Here's how the part is built. I have some questions about the finished solid (model axes, mm). A direction names the side the tool comes from. Round coordinates to 2 decimals unless told otherwise and drop trailing zeros. Loops run counter-clockwise (first coordinate to the right, second up) from the corner with the lowest first, then second, coordinate; pieces in that order, holes last. Notation, with made-up numbers: M 38.25,18 L 51.25,18 A33 ccw 51.25,54 Z; hole C -8,32 d7. An arc over 180 degrees is marked long. Answer as a JSON object with one key per item and string values.
Autodesk Inventor part; units mm, degrees
ref_plane "Work Plane1" through (-10, 2, -13) normal (1, 0, 0) x (0, 0, -1)
ref_plane "Work Plane2" through (0, 0, -6.5) normal (0, 0, -1) x (-1, 0, 0)
ref_plane "Work Plane3" through (0, 0, 0) normal (1, 0, 0) x (0, 0, -1)
sketch "Sketch1" plane through (0, 0, 0) normal (0, 1, 0) x (-1, 0, 0)
  line L0 (0, 0) -> (-20, 0)
  line L1 (-20, 0) -> (-20, -13)
  line L2 (-20, -13) -> (0, -13)
  line L3 (0, -13) -> (0, 0)
  line L4 (0, -13) -> (20, -13)
  line L5 (20, -13) -> (20, -10)
  line L6 (20, -10) -> (0, -10)
  line L7 (0, -10) -> (0, -13)
  line L8 (0, -13) -> (-20, -13)
  line L9 (-20, -13) -> (-20, -23)
  line L10 (-20, -23) -> (0, -23)
  line L11 (0, -23) -> (0, -13)
  line L12 (20, -10) -> (0, -10)
  line L13 (0, -10) -> (0, 0)
  line L14 (0, 0) -> (20, 0)
  line L15 (20, 0) -> (20, -10)
  dimension "d0" = 20
  dimension "d1" = 13
  dimension "d2" = 20
  dimension "d3" = 3
  dimension "d4" = 10
extrude "Extrusion1" add sketch "Sketch1" along normal blind 2 contours L3 L2 L1 L0 | L2 L11 L10 L9
extrude "Extrusion2" add sketch "Sketch1" along normal blind 22 contours L6 L5 L4 L3
extrude "Extrusion3" add sketch "Sketch1" along normal blind 2 contours L14 L15 L6 L3
ref_plane "Work Plane1" through (-10, 2, -13) normal (1, 0, 0) x (0, 0, -1)
sketch "Sketch2" plane through (-10, 2, -13) normal (1, 0, 0) x (0, 0, -1)
  line L0 (0, 20) -> (-3, 20)
  line L1 (-13, -2) -> (-13, 0)
  line L2 (-13, 0) -> (-3, 0)
  line L3 (-3, 0) -> (-3, 20)
  line L4 (-3, 0) -> (-3, 20)
  line L5 (-3, 20) -> (-13, 20)
  line L6 (-13, 20) -> (-13, 0)
  line L7 (-13, 0) -> (-3, 0)
  line L8 (-3, 0) -> (-3, 20)
extrude "Extrusion4" add sketch "Sketch2" along normal mid plane 20
fillet "Fillet1" radius 10 1 edges at (-10, 22, 0)
sketch "Sketch3" plane through (0, 0, -13) normal (0, 0, -1) x (-1, 0, 0)
  circle A0 centre (10, 16) radius 1.5
  line L0 (0, 22) -> (20, 22)
  circle A1 centre (10, 6) radius 1.5
  line L1 (0, 0) -> (20, 0)
  point P0 (10, 0)
  dimension "d14" = 3
  dimension "d15" = 6
  dimension "d16" = 3
  dimension "d18" = 6
extrude "Extrusion5" cut sketch "Sketch3" against normal blind 20
ref_plane "Work Plane2" through (0, 0, -6.5) normal (0, 0, -1) x (-1, 0, 0)
sketch "Sketch4" plane through (0, 0, -6.5) normal (0, 0, -1) x (-1, 0, 0)
  circle A0 centre (10, 16) radius 1.5
  circle A1 centre (10, 16) radius 3
  circle A2 centre (10, 6) radius 1.5
  circle A3 centre (10, 6) radius 3
  point P0 (0, 0)
  dimension "d21" = 6
  dimension "d22" = 6
extrude "Extrusion6" cut sketch "Sketch4" against normal blind 20
sketch "Sketch5" plane through (0, 0, -13) normal (0, 0, -1) x (-1, 0, 0)
  line L0 (0, 22) -> (20, 22)
  line L1 (0, 0) -> (20, 0)
  line L2 (0, 22) -> (20, 22)
  line L3 (20, 22) -> (20, 0)
  line L4 (20, 0) -> (0, 0)
  line L5 (0, 0) -> (0, 22)
  circle A0 centre (10, 16) radius 1.5
  circle A1 centre (10, 16) radius 1.5
  circle A2 centre (10, 6) radius 1.5
  circle A3 centre (10, 6) radius 1.5
extrude "Extrusion7" add sketch "Sketch5" along normal blind 10
ref_plane "Work Plane3" through (0, 0, 0) normal (1, 0, 0) x (0, 0, -1)
sketch "Sketch6" plane through (0, 0, 0) normal (1, 0, 0) x (0, 0, -1)
  line L0 (0, 0) -> (23, 0)
  line L1 (23, 0) -> (23, -2)
  line L2 (23, -2) -> (0, 0)
  line L3 (0, 0) -> (23, 0)
  dimension "d27" = 2
extrude "Extrusion8" add sketch "Sketch6" along normal mid plane 40
sketch "Sketch7" plane through (0, 22, -23) normal (0, 0, -1) x (-1, 0, 0)
  line L0 (20, 0) -> (0, 0)
  line L1 (20, -24) -> (20, -22)
  line L2 (0, 0) -> (20, 0)
  line L3 (20, 0) -> (20, -24)
  line L4 (20, -24) -> (0, -24)
  line L5 (0, -24) -> (0, 0)
  line L6 (0, -20) -> (-20, -20)
  line L7 (-20, -20) -> (0, -20)
  line L8 (0, -20) -> (0, -24)
  line L9 (0, -24) -> (-20, -24)
  line L10 (-20, -24) -> (-20, -20)
  circle A0 centre (10, -6) radius 1.5
  circle A1 centre (10, -6) radius 1.5
  circle A2 centre (10, -16) radius 1.5
  circle A3 centre (10, -16) radius 1.5
  point P0 (0, -22)
extrude "Extrusion9" add sketch "Sketch7" along normal blind 10
sketch "Sketch8" plane through (0, 0, 0) normal (1, 0, 0) x (0, 0, -1)
  line L0 (23, -2) -> (33, -2)
  line L1 (33, -2) -> (33, -3)
  line L2 (33, -3) -> (23, -2)
  point P0 (0, 0)
  dimension "d32" = 1
extrude "Extrusion10" add sketch "Sketch8" along normal mid plane 40
sketch "Sketch9" plane through (20, 0, 0) normal (1, 0, 0) x (0, 0, -1)
  line L0 (33, 2) -> (0, 2)
  line L1 (0, 2) -> (33, 2)
  line L2 (33, 2) -> (33, -3)
  line L3 (33, 2) -> (33, -3)
  line L4 (23, -2) -> (0, 0)
  line L5 (33, -3) -> (0, 0)
  line L6 (0, 0) -> (0, 2)
extrude "Extrusion11" add sketch "Sketch9" along normal blind 10
sketch "Sketch10" plane through (0, 22, -33) normal (0, 0, -1) x (-1, 0, 0)
  line L0 (0, -20) -> (-30, -20)
  line L1 (-30, -20) -> (0, -20)
  line L2 (0, -20) -> (0, -25)
  line L3 (-20, -25) -> (20, -25)
  line L4 (-30, -25) -> (-30, -20)
  line L5 (-30, -25) -> (-30, -20)
  line L6 (-20, -24) -> (-20, -25)
  line L7 (-20, -25) -> (-30, -25)
  line L8 (-20, -25) -> (-30, -25)
  point P0 (0, -22)
extrude "Extrusion12" add sketch "Sketch10" along normal blind 9
properties part number "Holder Motor Lifter 2"
Item 1: I want a section at B-B on y = 6. List the corners of the cut face in (x, z) for me, plus the area to 4 significant figures.
Solution:
{"outline": "M -20,-33 L -11.5,-33 L -11.5,-6.5 L -13,-6.5 L -13,0 L -20,0 Z; M -8.5,-33 L 0,-33 L 0,0 L -7,0 L -7,-6.5 L -8.5,-6.5 Z", "area": "541.5 mm2"}
Item 2: We'd pull the mould along Y, two halves only. Please class faces 4 (the face through (30, 0, -25)), 5 (the face through (-8.5, 15.93, -19.56)), 6 (the face through (-9.35, 13.07, -4.04)), 7 (the face through (24.93, -1.52, -16.73)): +Y half, -Y half, draft (parallel to the pull), parting line (faces both ways), or undercut.
Solution:
{"face 4": "draft", "face 5": "undercut", "face 6": "undercut", "face 7": "-Y half"}
Item 3: I want a section at A-A on z = -27.5. List the corners of the cut face in (x, y) for me.
Solution:
{"outline": "M -20,-2.45 L 20,-2.45 L 20,-2.5 L 30,-2.5 L 30,2 L 0,2 L 0,22 L -20,22 Z; hole C -10,6 d3; hole C -10,16 d3"}
Item 4: I want a section at D-D on x = -17. List the corners of the cut face in (y, z) for me, plus the area to 3 significant figures.
Solution:
{"outline": "M -3,-33 L 22,-33 L 22,-10 A10 ccw 12,0 L 0,0 L -2,-23 Z", "area": "753 mm2"}
Item 5: For faces 1 (the face through (15, 2, -21)), 2 (the face through (-11.3, 14.7, -6.5)), 3 (the face through (-10, 10, -33)), which set-ups out of +Z, -Z, +X, -X, +Y, -Y let a thin tool reach every point of the face, with its end or its side?
Solution:
{"face 1": "+Z, -Z, +X, +Y", "face 2": "+Z", "face 3": "-Z, -X, +Y, -Y"}
Item 6: I want a section at C-C on x = -10. List the corners of the cut face in (y, z) for me.
Solution:
{"outline": "M -3,-33 L 4.5,-33 L 4.5,-6.5 L 3,-6.5 L 3,0 L 0,0 L -2,-23 Z; M 7.5,-33 L 14.5,-33 L 14.5,-6.5 L 13,-6.5 L 13,-0.05 A10 ccw 12,0 L 9,0 L 9,-6.5 L 7.5,-6.5 Z; M 17.5,-33 L 22,-33 L 22,-10 A10 ccw 19,-2.86 L 19,-6.5 L 17.5,-6.5 Z"}
Item 7: For P1, Ø5, axis at x = -10, y = 16, coming from the -Z side; P2, Ø10, axis at y = 10.5, z = -8.5, coming from the +X side; P3, Ø3, axis at x = -8.5, z = -36, coming from the +Y side; P4, Ø5.5, axis at y = -1.5, z = -39.5, coming from the -X side, each with a flat end and sliding along its axis, tell me the tip position at first contact or that it passes through.
Solution:
{"P1": "stops at z = -33", "P2": "stops at x = 0", "P3": "passes through", "P4": "stops at x = 0"}
Item 8: If I drill on L1, parallel to Y at x = -10, z = -12.5; L2, parallel to Z at x = -3, y = 11.5; L3, parallel to X at y = 16, z = -4.75, over which ranges is the centre line in solid material (lowest first)? Write a range as from..to.
Solution:
{"L1": "y = -1.09..4.5, 7.5..14.5, 17.5..22", "L2": "z = -33..0", "L3": "x = -20..-13, -7..0"}
